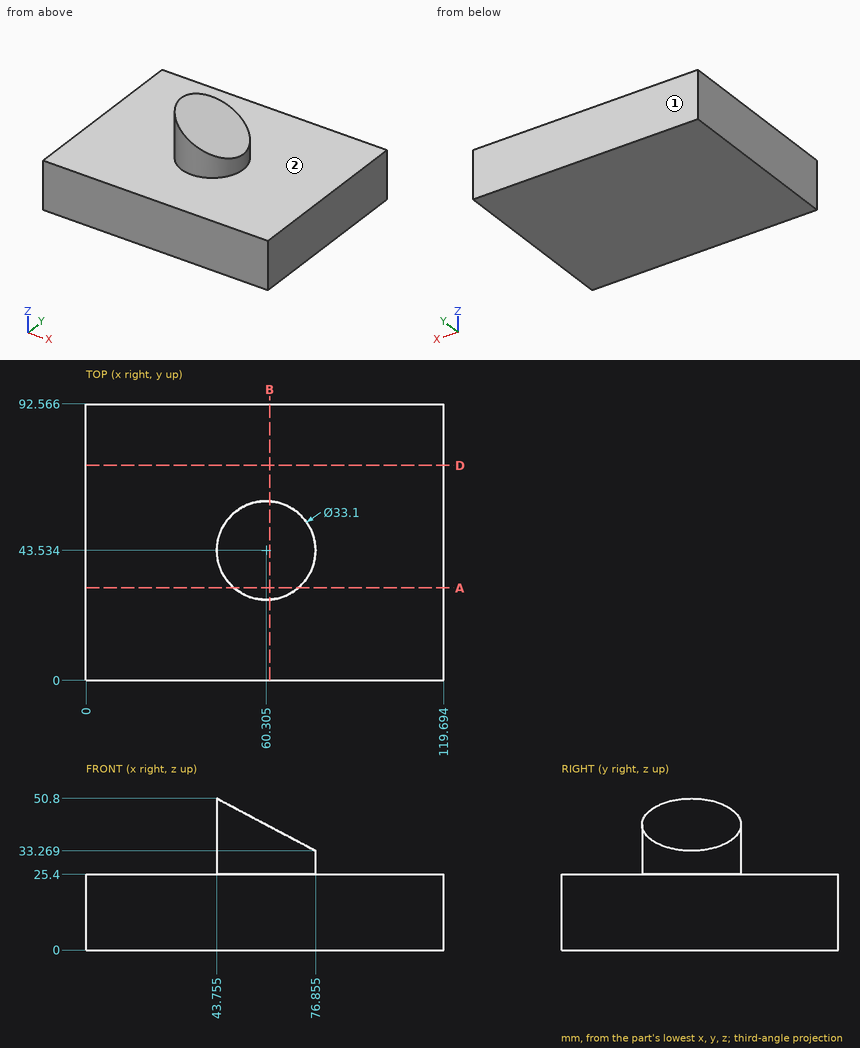
The drawing under review shows one solid part. Ordinate dimensions are in mm from its lowest x, y, z. A direction names the side the tool comes from. Round coordinates to 2 decimals unless told otherwise and drop trailing zeros. Write each loop counter-clockwise with the first axis right and the second up, starting at its lowest first coordinate (ties: lowest second). Pieces come first, ordered by that corner, then holes. Notation, with made-up numbers: M -6.5,69.5 L 11.5,69.5 A15 ccw 11.5,84.5 Z; hole C -23.75,-39 d4. An arc over 180 degrees is marked long. One line per item, written item: value. Start each with the question number.
(1) Wall thickness on line 1 (Z direction, x = 83, y = 22); line 2 (X direction, y = 39, z = 36) (1 decimal); line 3 (Z direction, x = 65.5, y = 43.5) (1 decimal): over which ranges is each line inside the solid? List them lowest first.
(2) Insertion check: pin 1 (3 mm diameter, centred on x = 101, z = 24, fed in from -Y); pin 2 (6 mm diameter, centred on y = 47, z = 32.5, fed in from -X); pin 3 (6 mm diameter, centred on x = 52, z = 37, fed in from -Y). Each pin has a flat end and moves straight along its axis. Give the tip position at first contact, or say it passes through.
(3) We need section B-B (x = 61.5). Give the boundary of the cut face in (y, z) (1 decimal).
(4) Machinability: for the marked faces 1 and 2, which of the approach directions +Z, -Z, +X, -X, +Y, -Y give a long, thin tool a straight path to every point of the face, cutting with its end or side? Answer none if there is none.
(5) We need section A-A (y = 31). Give the boundary of the cut face in (x, z) (1 decimal).
(6) We need section D-D (y = 72). Give the boundary of the cut face in (x, z) (1 decimal).
Result:
1. line 1: 0 to 25.4
1. line 2: 44.4 to 71.7
1. line 3: 0 to 39.3
2. pin 1: y = 0
2. pin 2: x = 43.76
2. pin 3: y = 27.86
3. outline: M 0,0 L 92.6,0 L 92.6,25.4 L 60,25.4 L 60,41.4 L 27,41.4 L 27,25.4 L 0,25.4 Z
4. face 1: +Z, -Z, +X, -X, +Y
4. face 2: +Z
5. outline: M 0,0 L 119.7,0 L 119.7,25.4 L 71.1,25.4 L 71.1,36.3 L 49.5,47.8 L 49.5,25.4 L 0,25.4 Z
6. outline: M 0,0 L 119.7,0 L 119.7,25.4 L 0,25.4 Z
